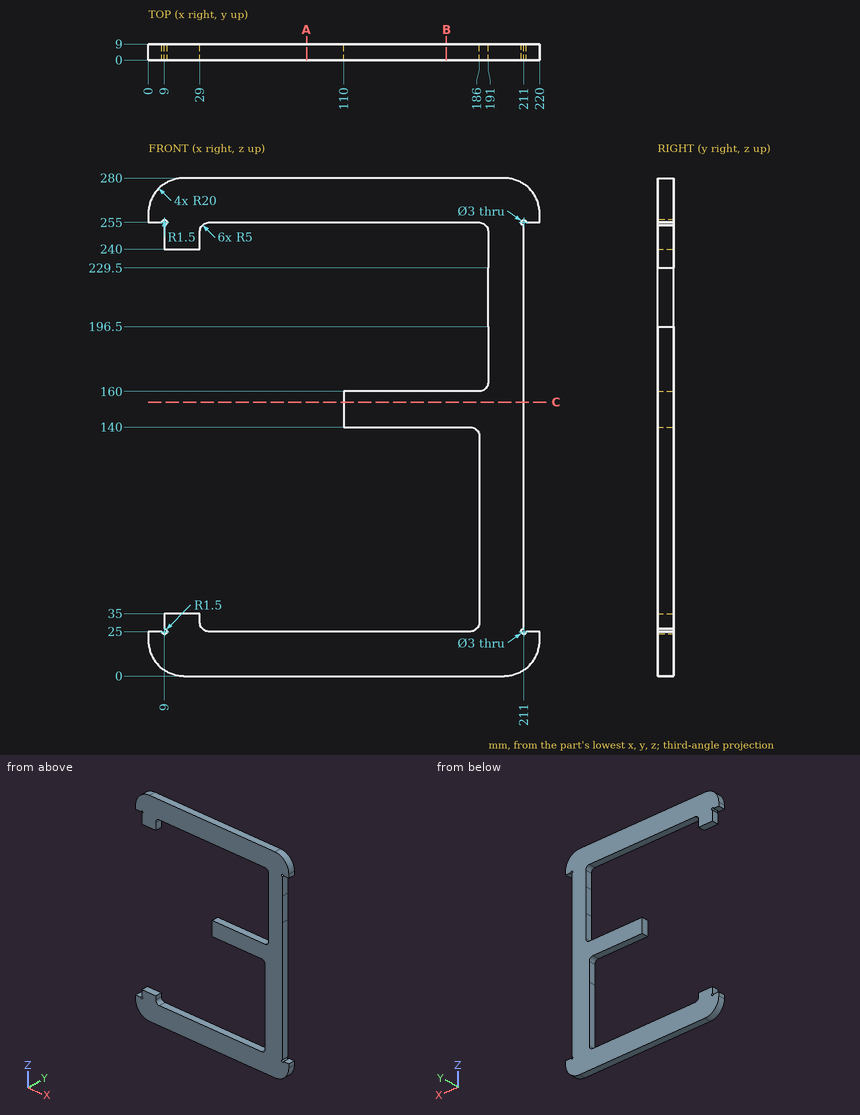
Can you work these out from the drawing? Everything is in mm from the part's minimum corner. Give positions to 0.01 mm unless a question says otherwise; leave off trailing zeros. Order: outer loops, then holes, each group sorted by start corner. A loop starts at its lowest first (then second) coordinate and runs counter-clockwise, first axis right, second up. Notation, with made-up numbers: M -23,67.5 L 10,67.5 A20 ccw 10,73.5 Z; hole C -21.75,57.25 d7. An arc over 180 degrees is marked long. One line per question, with ' | ' between items.
1. I want a section at A-A (x = 89). List the corners of the cut face in (y, z) for me.
Results:
outline: M 0,0 L 9,0 L 9,25 L 0,25 Z; M 0,255 L 9,255 L 9,280 L 0,280 Z
2. I want a section at B-B (x = 167.5). List the corners of the cut face in (y, z) for me.
Results:
outline: M 0,0 L 9,0 L 9,25 L 0,25 Z; M 0,140 L 9,140 L 9,160 L 0,160 Z; M 0,255 L 9,255 L 9,280 L 0,280 Z
3. I want a section at C-C (z = 154). List the corners of the cut face in (x, y) for me.
Results:
outline: M 110,0 L 211,0 L 211,9 L 110,9 Z
4. If I drill on line 1 (Z direction, x = 116, y = 1.25); line 2 (X direction, y = 7.5, z = 74); line 3 (X direction, y = 7, z = 27), over which ranges is the centre line in solid material (lowest first)?
Results:
line 1: 0 to 25, 140 to 160, 255 to 280 | line 2: 186 to 211 | line 3: 9 to 30, 185 to 211
5. I'm going to push flat-ended pins straight in: pin 1 (1.5 mm diameter, centred on y = 6, z = 233.5, fed in from +X); pin 2 (4.5 mm diameter, centred on y = 3.5, z = 213.5, fed in from -X); pin 3 (2.5 mm diameter, centred on y = 2.5, z = 32, fed in from -X). Where does each tip first touch, or does it pass through?
Results:
pin 1: x = 211 | pin 2: x = 191 | pin 3: x = 9
